```python
from build123d import *

# Parameters (mm, degrees)
SKETCH1_W           = 5
SKETCH1_H           = 30
BOSS_EXTRUDE1_DEPTH = 80
SKETCH2_R           = 1.2
SKETCH2_R_2         = 4.4
CUT_EXTRUDE1_DEPTH  = 80
CUT_EXTRUDE3_DEPTH  = 60
FILLET1_R           = 30
SKETCH6_R           = 10.5
SKETCH6_R_2         = 1.41450308
CUT_EXTRUDE4_DEPTH  = 151.748134317
SKETCH8_W           = 7
SKETCH8_H           = 29
CUT_EXTRUDE5_DEPTH  = 47


with BuildPart() as part:
    # Sketch1 → Boss-Extrude1 (new body)
    with BuildSketch(Plane.XY):
        Polygon((55, 35), (-55, 35), (-55, -35), (-24, -35), (-19, -35), (19, -35), (24, -35), (55, -35), align=None)
        with Locations((-21.5, -50)):
            Rectangle(SKETCH1_W, SKETCH1_H)
        with Locations((21.5, -50)):
            Rectangle(SKETCH1_W, SKETCH1_H)
    extrude(amount=BOSS_EXTRUDE1_DEPTH)

    # Sketch2 → Cut-Extrude1 (cut)
    with BuildSketch(Plane(origin=(24, 0, 0), x_dir=(0, 0, -1), z_dir=(1, 0, 0))):
        with Locations(Location((-40, -45, 0), (0, 0, 90))):
            Circle(SKETCH2_R)
        with Locations(Location((-32, -53, 0), (0, 0, 90))):
            Circle(SKETCH2_R)
        with Locations(Location((-40, -61, 0), (0, 0, 90))):
            Circle(SKETCH2_R)
        with Locations(Location((-48, -53, 0), (0, 0, 90))):
            Circle(SKETCH2_R)
        with Locations(Location((-40, -53, 0), (0, 0, 90))):
            Circle(SKETCH2_R_2)
    extrude(amount=-CUT_EXTRUDE1_DEPTH, mode=Mode.SUBTRACT)

    # Sketch4 → Cut-Extrude3 (cut)
    with BuildSketch(Plane(origin=(0, 35, 0), x_dir=(1, 0, 0), z_dir=(0, 1, 0))):
        Polygon((-45, 0), (-45, -80), (-15, -80), (-15, -60), (15, -60), (15, -80), (45, -80), (45, 0), (15, 0), (15, -5), (-15, -5), (-15, 0), align=None)
    extrude(amount=-CUT_EXTRUDE3_DEPTH, mode=Mode.SUBTRACT)

    # Fillet1
    fillet1_edges = [part.edges().sort_by_distance(p)[0] for p in [
        (-21.5, -65, 0),
        (-21.5, -65, 80),
        (21.5, -65, 0),
        (21.5, -65, 80),
    ]]
    fillet(fillet1_edges, radius=FILLET1_R)

    # Sketch6 → Cut-Extrude4 (cut, through all)
    with BuildSketch(Plane(origin=(55, 0, 0), x_dir=(0, 0, -1), z_dir=(1, 0, 0))):
        with Locations((-40, 23.75)):
            Circle(SKETCH6_R)
        with Locations((-51, 31.75)):
            Circle(SKETCH6_R_2)
        with Locations((-29, 31.75)):
            Circle(SKETCH6_R_2)
        with Locations((-51, -8.25)):
            Circle(SKETCH6_R_2)
        with Locations((-29, -8.25)):
            Circle(SKETCH6_R_2)
    extrude(amount=-CUT_EXTRUDE4_DEPTH, mode=Mode.SUBTRACT)

    # Sketch8 → Cut-Extrude5 (cut)
    with BuildSketch(Plane(origin=(0, 35, 0), x_dir=(1, 0, 0), z_dir=(0, 1, 0))):
        with Locations((-48.5, -40)):
            Rectangle(SKETCH8_W, SKETCH8_H)
        with Locations((48.5, -40)):
            Rectangle(SKETCH8_W, SKETCH8_H)
    extrude(amount=-CUT_EXTRUDE5_DEPTH, mode=Mode.SUBTRACT)


solid = part.part
```
Model file for the job. Use its own axes, mm. A direction names the side the tool comes from. Give positions to 0.01 mm unless a question says otherwise; leave off trailing zeros. Write each loop counter-clockwise with the first axis right and the second up, starting at its lowest first coordinate (ties: lowest second). Pieces come first, ordered by that corner, then holes. Notation, with made-up numbers: M 58,-35.75 L 72,-35.75 A22 cw 72,-26.75 Z; hole C -19.5,-33.75 d7. An arc over 180 degrees is marked long. Use a Markdown table: item, result.
1) Drill centre lines: line 1 (Y direction, x = -53, z = 51); line 2 (X direction, y = 1, z = 4); line 3 (X direction, y = -20.5, z = 11). Where is each one in solid material? Low to high. Write a range as from..to.
Responses:
| item | result |
|---|---|
| line 1 | y = -35..-9.66, -6.84..30.34, 33.16..35 |
| line 2 | x = -55..-45, -15..15, 45..55 |
| line 3 | x = -55..-45, 45..55 |
2) Pull direction X, two halves, no side cores. Call faces 4 (the flat face through (24, -47, 39)), 5 (the flat face through (-1, 0, 80)), 6 (the flat face through (-1, -25, 39)): +X half, -X half, draft (parallel to the pull), parting line (faces both ways), or undercut.
Responses:
| item | result |
|---|---|
| face 4 | +X half |
| face 5 | draft |
| face 6 | undercut |
3) Cut at C-C (y = 20.5). Give the number of separate pieces and of enclosed holes in the cut face, and give its area (3 significant figures).
Responses:
| item | result |
|---|---|
| separate pieces | 6 |
| enclosed holes | 0 |
| area | 1,820 mm2 |
4) Tool access for faces 1 (the flat face through (-22, -65, 40)), 2 (the flat face through (19, -47, 39)), 3 (the flat face through (-49, 12, 54.5)): list every direction of +Z, -Z, +X, -X, +Y, -Y with a clear straight run to the whole face (end or side of a thin tool).
Responses:
| item | result |
|---|---|
| face 1 | +Z, -Z, +X, -X, -Y |
| face 2 | +Z, -Z, -Y |
| face 3 | +Y |
5) Cut at B-B (x = -3.5). List the corners of the cut face in (y, z).
Responses:
| item | result |
|---|---|
| outline | M -35,0 L 35,0 L 35,5 L -25,5 L -25,60 L 35,60 L 35,80 L -35,80 Z |
6) Cut at A-A (y = -18). List the corners of the cut face in (x, z).
Responses:
| item | result |
|---|---|
| outline | M -55,0 L -45,0 L -45,80 L -55,80 Z; M -15,0 L 15,0 L 15,5 L -15,5 Z; M -15,60 L 15,60 L 15,80 L -15,80 Z; M 45,0 L 55,0 L 55,80 L 45,80 Z |
7) Cut at D-D (z = 8.5). List the corners of the cut face in (x, y).
Responses:
| item | result |
|---|---|
| outline | M -55,-35 L -24,-35 L -24,-55.92 L -19,-55.92 L -19,-35 L 19,-35 L 19,-55.92 L 24,-55.92 L 24,-35 L 55,-35 L 55,35 L 45,35 L 45,-25 L -45,-25 L -45,35 L -55,35 Z |
8) Pin check, flat tips, straight feed: pin 1 (14 mm diameter, centred on y = -53, z = 40, fed in from +X); pin 2 (10 mm diameter, centred on y = -53, z = 40, fed in from -X); pin 3 (2.5 mm diameter, centred on y = -8.25, z = 51, fed in from -X); pin 4 (4 mm diameter, centred on x = 20, y = -51, fed in from +Z). Stop position of each tip, or through.
Responses:
| item | result |
|---|---|
| pin 1 | stops at x = 24 |
| pin 2 | stops at x = -24 |
| pin 3 | passes through |
| pin 4 | stops at z = 76.53 |
